from build123d import *

# Parameters (mm, degrees)
SKETCH1_R                        = 6.5405
SKETCH1_R_2                      = 2.9845
BOSS_EXTRUDE1_DEPTH              = 4.826
SKETCH2_R                        = 2.032
BOSS_EXTRUDE2_DEPTH              = 4.826
F_42_0_0935_DIAMETER_HOLE1_D     = 2.3749
F_42_0_0935_DIAMETER_HOLE1_DEPTH = 2.032
F_42_0_0935_DIAMETER_HOLE1_TIP   = 0.713491942
BOSS_EXTRUDE3_DEPTH              = 4.826
CUT_EXTRUDE1_DEPTH               = 2.50825
CUT_EXTRUDE2_DEPTH               = 5.826
LPATTERN1_COUNT                  = 14
LPATTERN1_PITCH                  = 0.7874
CUT_EXTRUDE3_DEPTH               = 5.826
CIRPATTERN1_COUNT                = 13
CIRPATTERN1_ANGLE                = 76.5
SKETCH13_W                       = 4.953
SKETCH13_H                       = 2.54
CUT_EXTRUDE5_DEPTH               = 2.50825
BOSS_EXTRUDE4_REACH              = 28.099
SKETCH15_W                       = 4.953
SKETCH15_H                       = 2.54
CUT_EXTRUDE6_DEPTH               = 2.50825
SKETCH16_R                       = 6.5405
CUT_EXTRUDE7_DEPTH               = 2.54


with BuildPart() as part:
    # Sketch1 → Boss-Extrude1 (new body)
    with BuildSketch(Plane(origin=(0, 0, 0), x_dir=(1, 0, 0), z_dir=(0, 1, 0))):
        Circle(SKETCH1_R)
        Circle(SKETCH1_R_2, mode=Mode.SUBTRACT)
    extrude(amount=BOSS_EXTRUDE1_DEPTH)

    # Sketch2 → Boss-Extrude2 (add)
    with BuildSketch(Plane(origin=(0, 0, 0), x_dir=(1, 0, 0), z_dir=(0, 1, 0))):
        with BuildLine():
            Line((-6.5405, 0), (-13.5255, 0))
            Line((-13.5255, 0), (-13.5255, -2.137742196))
            Line((-13.5255, -2.137742196), (-15.655107442, -1.951425687))
            ThreePointArc((-15.655107442, -1.951425687), (-20.569516848, -6.947096437), (-14.732, -10.824149842))
            Line((-14.732, -10.824149842), (-0.540673648, -6.518114164))
            ThreePointArc((-0.540673648, -6.518114164), (-4.812193691, -4.429552136), (-6.5405, 0))
        make_face()
        with Locations((-16.05104389, -6.477)):
            Circle(SKETCH2_R, mode=Mode.SUBTRACT)
    extrude(amount=BOSS_EXTRUDE2_DEPTH)

    # #42 (0.0935) Diameter Hole1
    with Locations(Plane(origin=(0, 0, 0), x_dir=(-1, 0, 0), z_dir=(0, 0, -1))):
        with Locations((10.033, 2.413)):
            Hole(F_42_0_0935_DIAMETER_HOLE1_D / 2, depth=F_42_0_0935_DIAMETER_HOLE1_DEPTH)
            with Locations((0, 0, -(F_42_0_0935_DIAMETER_HOLE1_DEPTH + F_42_0_0935_DIAMETER_HOLE1_TIP / 2))):  # 118° drill point
                Cone(0, F_42_0_0935_DIAMETER_HOLE1_D / 2, F_42_0_0935_DIAMETER_HOLE1_TIP, mode=Mode.SUBTRACT)

    # Sketch8 → Boss-Extrude3 (add)
    with BuildSketch(Plane(origin=(0, 0, 0), x_dir=(1, 0, 0), z_dir=(0, 1, 0))):
        with BuildLine():
            Line((13.001568547, 6.9215), (32.639, 1.524))
            Line((32.639, 1.524), (32.639, 0))
            Line((32.639, 0), (21.5265, 0))
            ThreePointArc((21.5265, 0), (16.51, 1.884223876), (11.4935, 0))
            Line((11.4935, 0), (6.5405, 0))
            ThreePointArc((6.5405, 0), (5.703778696, 3.200788783), (3.407697053, 5.582628507))
            Line((3.407697053, 5.582628507), (4.746568547, 6.9215))
            Line((4.746568547, 6.9215), (13.001568547, 6.9215))
        make_face()
    extrude(amount=BOSS_EXTRUDE3_DEPTH)

    # Sketch9 → Cut-Extrude1 (cut)
    with BuildSketch(Plane(origin=(0, 4.826, 0), x_dir=(1, 0, 0), z_dir=(0, 1, 0))):
        with BuildLine():
            ThreePointArc((-7.3025, 0), (-5.860688184, -4.356471079), (-2.10459784, -6.992651442))
            Line((-2.10459784, -6.992651442), (-0.540673648, -6.518114164))
            ThreePointArc((-0.540673648, -6.518114164), (-4.812193691, -4.429552136), (-6.5405, 0))
            Line((-6.5405, 0), (-7.3025, 0))
        make_face()
    extrude(amount=-CUT_EXTRUDE1_DEPTH, mode=Mode.SUBTRACT)

    # Sketch10 → Cut-Extrude2 (cut, through all)
    with BuildSketch(Plane(origin=(0, 4.826, 0), x_dir=(1, 0, 0), z_dir=(0, 1, 0))):
        Polygon((32.639, 0), (32.258, 0.381), (31.877, 0), align=None)
    cut_extrude2 = extrude(amount=-CUT_EXTRUDE2_DEPTH, mode=Mode.SUBTRACT)

    # LPattern1: Cut-Extrude2 ×14
    with Locations(*[(-i * LPATTERN1_PITCH, 0, 0) for i in range(1, LPATTERN1_COUNT)]):
        add(cut_extrude2, mode=Mode.SUBTRACT)

    # Sketch11 → Cut-Extrude3 (cut, through all)
    with BuildSketch(Plane(origin=(0, 4.826, 0), x_dir=(1, 0, 0), z_dir=(0, 1, 0))):
        with BuildLine():
            Line((21.5265, 0), (21.464606941, 0.546569859))
            Line((21.464606941, 0.546569859), (20.918663717, 0.47937345))
            ThreePointArc((20.918663717, 0.47937345), (21.228673277, 0.247410527), (21.5265, 0))
        make_face()
    cut_extrude3 = extrude(amount=-CUT_EXTRUDE3_DEPTH, mode=Mode.SUBTRACT)

    # CirPattern1: Cut-Extrude3 ×13 about axis
    cirpattern1_axis = Axis((16.51, 0, 5.735776124), (0, 1, 0))
    for i in range(1, CIRPATTERN1_COUNT):
        add(cut_extrude3.rotate(cirpattern1_axis, i * CIRPATTERN1_ANGLE / (CIRPATTERN1_COUNT - 1)), mode=Mode.SUBTRACT)

    # Sketch13 → Cut-Extrude5 (cut)
    with BuildSketch(Plane(origin=(0, 4.826, 0), x_dir=(1, 0, 0), z_dir=(0, 1, 0))):
        with Locations((9.017, 1.27)):
            Rectangle(SKETCH13_W, SKETCH13_H)
    extrude(amount=-CUT_EXTRUDE5_DEPTH, mode=Mode.SUBTRACT)

    # Sketch14 → Boss-Extrude4 (add, up to next)
    with BuildSketch(Plane(origin=(6.5405, 0, 0), x_dir=(0, 0, -1), z_dir=(1, 0, 0)), mode=Mode.PRIVATE) as boss_extrude4_sk1:
        Polygon((0, 2.31775), (2.54, 4.826), (2.54, 2.31775), align=None)
    boss_extrude4_tool1 = extrude(boss_extrude4_sk1.sketch, amount=BOSS_EXTRUDE4_REACH, mode=Mode.PRIVATE) - part.part
    add(boss_extrude4_tool1.solids().sort_by_distance((6.5405, 3.153833, -1.693333))[0])

    # Sketch15 → Cut-Extrude6 (cut)
    with BuildSketch(Plane.XZ):
        with Locations((9.017, -1.27)):
            Rectangle(SKETCH15_W, SKETCH15_H)
    extrude(amount=-CUT_EXTRUDE6_DEPTH, mode=Mode.SUBTRACT)

    # Sketch16 → Cut-Extrude7 (cut)
    with BuildSketch(Plane(origin=(0, 4.826, 0), x_dir=(1, 0, 0), z_dir=(0, 1, 0))):
        Circle(SKETCH16_R)
    extrude(amount=-CUT_EXTRUDE7_DEPTH, mode=Mode.SUBTRACT)


solid = part.part
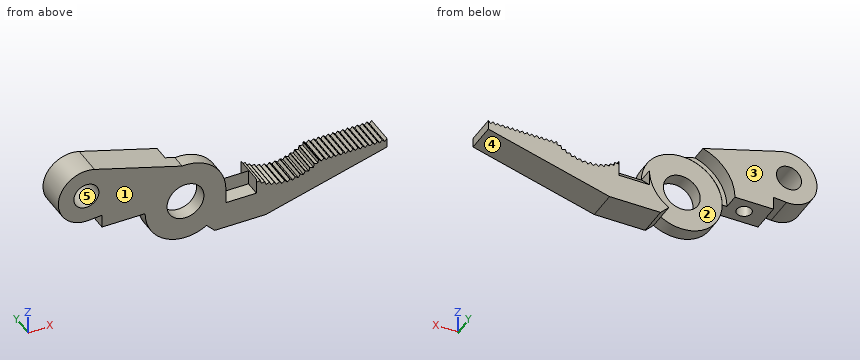
Design review of the part built by this model. Coordinates are the model's own, in mm. Face numbers are marked on the shaded views. A direction names the side the tool comes from. Round coordinates to 2 decimals unless told otherwise and drop trailing zeros. Write each loop counter-clockwise with the first axis right and the second up, starting at its lowest first coordinate (ties: lowest second). Pieces come first, ordered by that corner, then holes. Notation, with made-up numbers: (-33.75, 53.25) - (3.25, 53.25) arc R20 cw to (3.25, 65.25) - close; hole circle Ø11 at (71.25, 2). An arc over 180 degrees is marked (long way). Return JSON: item names as keys, results as strings. Group by question number.
Item 1: Machinability: for the marked faces 1 and 2, which of the approach directions +Z, -Z, +X, -X, +Y, -Y give a long, thin tool a straight path to every point of the face, cutting with its end or side? Answer none if there is none.
Item 2: We need section C-C on x = 10.5. Write out the cut boundary in (y, z).
Item 3: Insertion check: P1, Ø4, axis at x = -1, z = 1.5, coming from the +Y side; P2, Ø0.7, axis at x = 8, z = -1, coming from the -Y side; P3, Ø2.5, axis at x = -11.5, y = 3.5, coming from the -Z side. Each pin has a flat end and moves straight along its axis. Give the tip position at first contact, or say it passes through.
Item 4: For probe 1 along Z at (x, y) = (0, 1.7); probe 2 along Z at (x, y) = (30.5, 0.4); probe 3 along X at (y, z) = (0.65, 2.75), list the stretches that pass through material, from the lowest coordinate up. Write a range as [from, to].
Item 5: We need section A-A on x = 0. Write out the cut boundary in (y, z).
Item 6: The part is to be moulded in two halves that separate along X. For the marked faces 3, 4 and 5, say which applies: pulls with the +X half, pulls with the -X half, needs draft (parallel to the pull), parting line crosses it, or undercut.
Model answer:
{
 "1": {"face 1": "+Z, -Z, +X, -X, -Y", "face 2": "+Y"},
 "2": {"outline": "(0, -6.92) - (4.83, -6.92) - (4.83, -2.54) - (2.51, -0.19) - (2.51, -2.54) - (0, -2.54) - close"},
 "3": {"P1": "stops at y = 2.29", "P2": "stops at y = 2.51", "P3": "stops at z = 0"},
 "4": {"probe 1": "z = [-6.54, -2.98], [2.98, 6.54]", "probe 2": "z = [-2.11, -0.2]", "probe 3": "x = [-18.65, -1.16], [1.16, 5.93]"},
 "5": {"outline": "(0, -6.54) - (2.29, -6.54) - (2.29, -2.98) - (0, -2.98) - close; (0, 2.98) - (2.29, 2.98) - (2.29, 6.54) - (0, 6.54) - close"},
 "6": {"face 3": "needs draft", "face 4": "pulls with the +X half", "face 5": "undercut"}
}
